```python
from build123d import *

# Parameters (mm, degrees)
F1_DEPTH = 10
F3_DEPTH = 7.5
F5_DEPTH = 25
F8_DEPTH = 2.2


with BuildPart() as f1:
    # F0 (on Top) → F1 (new body)
    with BuildSketch(Plane.XY):
        with BuildLine():
            Line((-4.6041666667, 7.1450436881), (-6.5, 10.0871205009))
            ThreePointArc((-6.5, 10.0871205009), (0, -12), (6.5, 10.0871205009))
            Line((6.5, 10.0871205009), (4.6041666667, 7.1450436881))
            ThreePointArc((4.6041666667, 7.1450436881), (0, 8.5), (-4.6041666667, 7.1450436881))
        make_face()
        with BuildLine():
            ThreePointArc((-1.05, 1.2727922061), (1.65, 0), (-1.05, -1.2727922061))
            Line((-1.05, -1.2727922061), (-1.05, 1.2727922061))
        make_face(mode=Mode.SUBTRACT)
    extrude(amount=F1_DEPTH)

    # F2 (on Top) → F3 (cut)
    with BuildSketch(Plane.XY):
        Polygon((-4, 0), (-4, 3.1), (-6.8, 3.1), (-6.8, -3.1), (-4, -3.1), align=None)
    extrude(amount=F3_DEPTH, mode=Mode.SUBTRACT)

    # F4 (on Right) → F5 (cut)
    with BuildSketch(Plane.YZ):
        with BuildLine():
            ThreePointArc((0, 1.4), (1.1313708499, 1.8686291501), (1.6, 3))
            ThreePointArc((1.6, 3), (-1.1313708499, 4.1313708499), (0, 1.4))
        make_face()
    extrude(amount=-F5_DEPTH, mode=Mode.SUBTRACT)

    # F7 (on offset) → F8 (cut)
    with BuildSketch(Plane(origin=(-12, 0, 0), x_dir=(0, -1, 0), z_dir=(-1, 0, 0))):
        with BuildLine():
            Line((3, -2.9697169084), (3, 3))
            ThreePointArc((3, 3), (0, 6), (-3, 3))
            Line((-3, 3), (-3, -2.9697169084))
            Line((-3, -2.9697169084), (3, -2.9697169084))
        make_face()
    extrude(amount=-F8_DEPTH, mode=Mode.SUBTRACT)


solid = f1.part
```
Source: CAD feature listing. Evaluate the final solid. Frame: model axes, mm. A direction names the side the tool comes from. Round coordinates to 2 decimals unless told otherwise and drop trailing zeros. Loops run counter-clockwise (first coordinate to the right, second up) from the corner with the lowest first, then second, coordinate; pieces in that order, holes last.
1. Section query A-A on z = 6.5. Output: boundary loops of the cut face in (x, y).
2. Section query C-C on y = 0.5. Output: boundary loops of the cut face in (x, z).
3. Ray query, L1, parallel to Z at x = -3.25, y = 0; L2, parallel to Y at x = 0, z = 4.25; L3, parallel to Z at x = -6.75, y = -2. Return the intervals inside material, ascending.
4. Contact query for flat-ended pins moving along their axis: pin 1 (1.8 mm diameter, centred on y = -1, z = 3.5, fed in from -X); pin 2 (5 mm diameter, centred on y = 7, z = 8.5, fed in from -X); pin 3 (4 mm diameter, centred on y = 3, z = 9, fed in from +X). Output: stop coordinate, or through.
5. Section query B-B on x = 0. Output: boundary loops of the cut face in (y, z).
6. Mould query, pull axis Y, two halves, no side actions, for faces 5 (the flat face through (-5, -3.1, 4)), 6 (the flat face through (0, -3, 0)), 7 (the cylindrical face through (0, -12, 5)). Classes: released by +Y, released by -Y, zero draft, split by the parting line, or undercut.
7. Section query D-D on z = 8.5. Output: boundary loops of the cut face in (x, y).
8. Access query for faces 1 (the flat face through (-1.05, 0, 1)), 2 (the cylindrical face through (-11, 0, 6)), 3 (the flat face through (-4, -1, 5)), 4 (the flat face through (5.565, 8.637, 4.93)). Directions: +Z, -Z, +X, -X, +Y, -Y. A direction counts if a zero-diameter tool reaches every point of the face in a straight line with its end or side. Return the directions, or none.
Answers below:
1. outline: (-6.5, 10.09) arc R12 ccw (long way) to (6.5, 10.09) - (4.6, 7.15) arc R8.5 ccw to (-4.6, 7.15) - close; hole (-6.8, -3.1) - (-4, -3.1) - (-4, 3.1) - (-6.8, 3.1) - close; hole (-1.05, -1.27) arc R1.65 ccw (long way) to (-1.05, 1.27) - close
2. outline: (-11.99, 5.96) - (-9.8, 5.96) - (-9.8, 4.52) - (-6.8, 4.52) - (-6.8, 7.5) - (-4, 7.5) - (-4, 4.52) - (-1.05, 4.52) - (-1.05, 10) - (-11.99, 10) - close; (-9.8, 0) - (-6.8, 0) - (-6.8, 1.48) - (-9.8, 1.48) - close; (-4, 0) - (-1.05, 0) - (-1.05, 1.48) - (-4, 1.48) - close; (1.57, 0) - (11.99, 0) - (11.99, 10) - (1.57, 10) - close
3. L1: z = 0 to 1.4, 4.6 to 10
3. L2: y = -12 to -1.65, 1.65 to 8.5
3. L3: z = 7.5 to 10
4. pin 1: stops at x = -9.8
4. pin 2: stops at x = -11.12
4. pin 3: stops at x = 11.96
5. outline: (-12, 0) - (-1.65, 0) - (-1.65, 10) - (-12, 10) - close; (1.65, 0) - (8.5, 0) - (8.5, 10) - (1.65, 10) - close
6. face 5: undercut
6. face 6: zero draft
6. face 7: split by the parting line
7. outline: (-6.5, 10.09) arc R12 ccw (long way) to (6.5, 10.09) - (4.6, 7.15) arc R8.5 ccw to (-4.6, 7.15) - close; hole (-1.05, -1.27) arc R1.65 ccw (long way) to (-1.05, 1.27) - close
8. face 1: +Z, -Z
8. face 2: -Z, -X
8. face 3: -Z
8. face 4: +Z, -Z, +Y
